Source: CAD feature listing. Evaluate the final solid. Frame: model axes, mm. Give positions to 0.01 mm unless a question says otherwise; leave off trailing zeros. Write each loop counter-clockwise with the first axis right and the second up, starting at its lowest first coordinate (ties: lowest second). Pieces come first, ordered by that corner, then holes. Notation, with made-up numbers: M 34.5,27.5 L 39.5,27.5 A14 cw 39.5,51.5 Z; hole C -20.75,83 d2. An arc over 180 degrees is marked long. Return JSON: item names as keys, results as strings.
```python
from build123d import *

# Parameters (mm, degrees)
SKETCH1_R           = 1.5
BOSS_EXTRUDE1_DEPTH = 1.3
SKETCH2_R           = 16.25
SKETCH2_R_2         = 1.25
CUT_EXTRUDE1_DEPTH  = 1.3


with BuildPart() as part:
    # Sketch1 → Boss-Extrude1 (new body)
    with BuildSketch(Plane(origin=(0, 0, 0), x_dir=(1, 0, 0), z_dir=(0, 1, 0))):
        with BuildLine():
            Line((-56, -42), (56, -42))
            ThreePointArc((56, -42), (58.828427125, -40.828427125), (60, -38))
            Line((60, -38), (60, 38))
            ThreePointArc((60, 38), (58.828427125, 40.828427125), (56, 42))
            Line((56, 42), (-56, 42))
            ThreePointArc((-56, 42), (-58.828427125, 40.828427125), (-60, 38))
            Line((-60, 38), (-60, -38))
            ThreePointArc((-60, -38), (-58.828427125, -40.828427125), (-56, -42))
        make_face()
        with Locations((-56, 38)):
            Circle(SKETCH1_R, mode=Mode.SUBTRACT)
        with Locations((56, 38)):
            Circle(SKETCH1_R, mode=Mode.SUBTRACT)
        with Locations((56, -38)):
            Circle(SKETCH1_R, mode=Mode.SUBTRACT)
        with Locations((-56, -38)):
            Circle(SKETCH1_R, mode=Mode.SUBTRACT)
    extrude(amount=BOSS_EXTRUDE1_DEPTH)

    # Sketch2 → Cut-Extrude1 (cut)
    with BuildSketch(Plane(origin=(0, 1.3, 0), x_dir=(1, 0, 0), z_dir=(0, 1, 0))):
        with Locations((0, 9.5)):
            Circle(SKETCH2_R)
        with Locations((-49, -35)):
            Circle(SKETCH2_R_2)
        with Locations((-39, -35)):
            Circle(SKETCH2_R_2)
        with BuildLine():
            Line((-49, 22), (-49, -22))
            ThreePointArc((-49, -22), (-45, -26), (-41, -22))
            Line((-41, -22), (-41, 22))
            ThreePointArc((-41, 22), (-45, 26), (-49, 22))
        make_face()
        with BuildLine():
            Line((49, 22), (49, -22))
            ThreePointArc((49, -22), (45, -26), (41, -22))
            Line((41, -22), (41, 22))
            ThreePointArc((41, 22), (45, 26), (49, 22))
        make_face()
    extrude(amount=-CUT_EXTRUDE1_DEPTH, mode=Mode.SUBTRACT)


solid = part.part
```
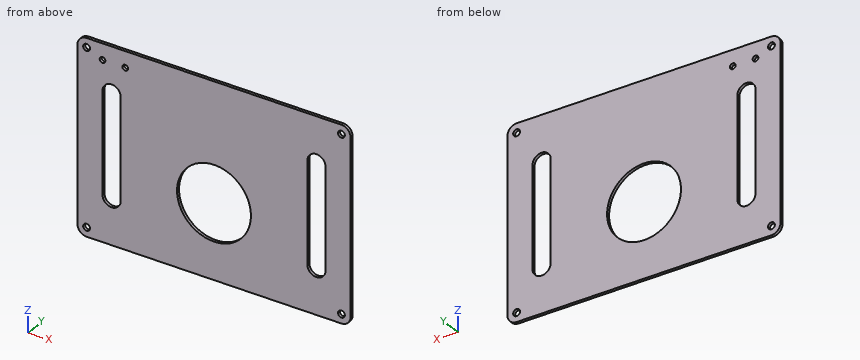
1) Contact query for a flat-ended pin moving along its axis: pin 1 Ø1.5 at (x, z) = (-0.5, 22.5) entering from -Y. Output: stop coordinate, or through.
Numbers:
{"pin 1": "stops at y = 0"}
2) Cut plane A-A, the plane x = 0. Return the cut outline in (y, z).
Numbers:
{"outline": "M 0,-42 L 1.3,-42 L 1.3,-25.75 L 0,-25.75 Z; M 0,6.75 L 1.3,6.75 L 1.3,42 L 0,42 Z"}
3) Cut plane D-D, the plane z = 35. Return the cut outline in (x, y), then the cut area to 4 significant figures.
Numbers:
{"outline": "M -60,0 L -50.25,0 L -50.25,1.3 L -60,1.3 Z; M -47.75,0 L -40.25,0 L -40.25,1.3 L -47.75,1.3 Z; M -37.75,0 L 60,0 L 60,1.3 L -37.75,1.3 Z", "area": "149.5 mm²"}
4) Cut plane B-B, the plane z = -13.5. Return the cut outline in (x, y), then the cut area to 4 significant figures.
Numbers:
{"outline": "M -60,0 L -49,0 L -49,1.3 L -60,1.3 Z; M -41,0 L -15.75,0 L -15.75,1.3 L -41,1.3 Z; M 15.75,0 L 41,0 L 41,1.3 L 15.75,1.3 Z; M 49,0 L 60,0 L 60,1.3 L 49,1.3 Z", "area": "94.25 mm²"}
5) Cut plane C-C, the plane y = 0.5. Give the number of separate pieces and of enclosed holes in the cut face, then the cut area to 3 significant figures.
Numbers:
{"separate pieces": "1", "enclosed holes": "9", "area": "8,390 mm²"}
6) Line query: line 1 (Z direction, x = 56, y = 0.5); line 2 (X direction, y = 0.6, z = 38); line 3 (X direction, y = 0.7, z = -9.5). Output: solid intervals per line, ascending. Write a range as [from, to].
Numbers:
{"line 1": "z = [-42, -39.5], [-36.5, 36.5], [39.5, 42]", "line 2": "x = [-60, -57.5], [-54.5, 54.5], [57.5, 60]", "line 3": "x = [-60, -49], [-41, -16.25], [16.25, 41], [49, 60]"}
